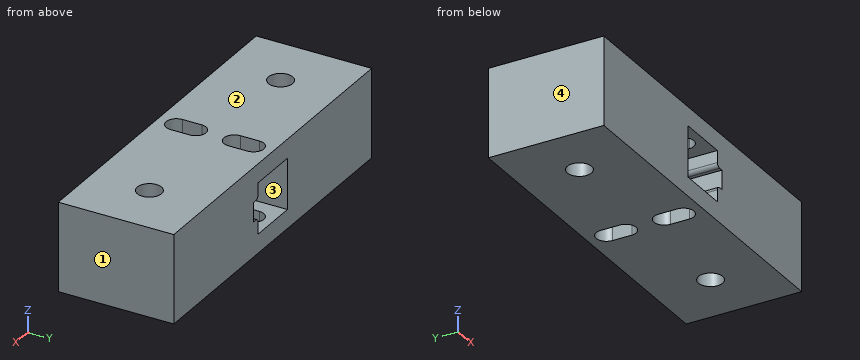
```python
from build123d import *

# Parameters (mm, degrees)
ESQUISSE1_W             = 89
ESQUISSE1_H             = 30
BOSS_EXTRU_1_DEPTH      = 23
ESQUISSE2_W             = 13.2
ESQUISSE2_H             = 13.2
ESQUISSE2_W_2           = 2
ESQUISSE2_H_2           = 5
ENL_V_MAT_EXTRU_1_DEPTH = 31
ESQUISSE3_R             = 3.15
ENL_V_MAT_EXTRU_2_DEPTH = 24
ENL_V_MAT_EXTRU_3_DEPTH = 24
CONG_1_R                = 1


with BuildPart() as part:
    # Esquisse1 → Boss.-Extru.1 (new body)
    with BuildSketch(Plane.XY):
        with Locations((40.389968792, -13.091136671)):
            Rectangle(ESQUISSE1_W, ESQUISSE1_H)
    extrude(amount=BOSS_EXTRU_1_DEPTH)

    # Esquisse2 → Enlèv. mat.-Extru.1 (cut, through all)
    with BuildSketch(Plane(origin=(0, 1.908863329, 0), x_dir=(1, 0, 0), z_dir=(0, 1, 0))):
        with Locations((40.389968792, -11.5)):
            Rectangle(ESQUISSE2_W, ESQUISSE2_H)
        with Locations((47.989968792, -11.5)):
            Rectangle(ESQUISSE2_W_2, ESQUISSE2_H_2)
    extrude(amount=-ENL_V_MAT_EXTRU_1_DEPTH, mode=Mode.SUBTRACT)

    # Esquisse3 → Enlèv. mat.-Extru.2 (cut, through all)
    with BuildSketch(Plane(origin=(0, 0, 0), x_dir=(-1, 0, 0), z_dir=(0, 0, -1))):
        with Locations((-10.889968792, -13.091136671)):
            Circle(ESQUISSE3_R)
        with Locations((-69.889968792, -13.091136671)):
            Circle(ESQUISSE3_R)
    extrude(amount=-ENL_V_MAT_EXTRU_2_DEPTH, mode=Mode.SUBTRACT)

    # Esquisse4 → Enlèv. mat.-Extru.3 (cut, through all)
    with BuildSketch(Plane(origin=(0, 0, 0), x_dir=(-1, 0, 0), z_dir=(0, 0, -1))):
        with BuildLine():
            ThreePointArc((-37.689968792, -8.091136671), (-40.389968792, -10.791136671), (-43.089968792, -8.091136671))
            Line((-43.089968792, -8.091136671), (-43.089968792, -3.091136671))
            ThreePointArc((-43.089968792, -3.091136671), (-40.389968792, -0.391136671), (-37.689968792, -3.091136671))
            Line((-37.689968792, -3.091136671), (-37.689968792, -8.091136671))
        make_face()
        with BuildLine():
            Line((-43.089968792, -23.091136671), (-43.089968792, -18.091136671))
            ThreePointArc((-43.089968792, -18.091136671), (-40.389968792, -15.391136671), (-37.689968792, -18.091136671))
            Line((-37.689968792, -18.091136671), (-37.689968792, -23.091136671))
            ThreePointArc((-37.689968792, -23.091136671), (-40.389968792, -25.791136671), (-43.089968792, -23.091136671))
        make_face()
    extrude(amount=-ENL_V_MAT_EXTRU_3_DEPTH, mode=Mode.SUBTRACT)

    # Congé1
    cong_1_edges = [part.edges().sort_by_distance(p)[0] for p in [
        (46.989968792, -13.091136671, 9),
        (46.989968792, -13.091136671, 14),
    ]]
    fillet(cong_1_edges, radius=CONG_1_R)


solid = part.part
```
Work out the finished part from the listing and answer in its coordinate system (mm). Face numbers are marked on the shaded views. Give positions to 0.01 mm unless a question says otherwise; leave off trailing zeros. Order: outer loops, then holes, each group sorted by start corner. A loop starts at its lowest first (then second) coordinate and runs counter-clockwise, first axis right, second up. Notation, with made-up numbers: (3.5, 54) - (52.5, 54) arc R8 ccw to (52.5, 62) - close; hole circle Ø8 at (25, 43.5). An arc over 180 degrees is marked (long way). One line per item, written item: value. Start each with the question number.
1. Section D-D, the plane x = 70.5 is taken. Write down the section's boundary in (y, z).
2. Section B-B, the plane x = 38.5 is taken. Write down the section's boundary in (y, z).
3. Each of these flat-tipped pins is pushed along its axis until it touches: pin 1 Ø5 at (x, y) = (10.89, -13.09) entering from +Z; pin 2 Ø10 at (x, y) = (59, -1.5) entering from -Z. Where does it stop, or does it pass through?
4. Consider line 1 (X direction, y = -12.75, z = 18.5); line 2 (X direction, y = -6, z = 2); line 3 (X direction, y = -13.25, z = 10.5). Determine where each line is inside the solid, lowest interval first.
5. Section C-C, the plane z = 10 is taken. Write down the section's boundary in (x, y).
6. Section A-A, the plane y = -20.75 is taken. Write down the section's boundary in (x, z).
7. For a pull along X with two mould halves and no side action, classify the marked faces 1, 2, 3 and 4 as released by +X, released by -X, zero draft, split by the parting line, or undercut.
Filled sheet:
1. outline: (-28.09, 0) - (-16.18, 0) - (-16.18, 23) - (-28.09, 23) - close; (-10, 0) - (1.91, 0) - (1.91, 23) - (-10, 23) - close
2. outline: (-28.09, 0) - (-25.02, 0) - (-25.02, 4.9) - (-28.09, 4.9) - close; (-28.09, 18.1) - (-25.02, 18.1) - (-25.02, 23) - (-28.09, 23) - close; (-16.16, 0) - (-10.02, 0) - (-10.02, 4.9) - (-16.16, 4.9) - close; (-16.16, 18.1) - (-10.02, 18.1) - (-10.02, 23) - (-16.16, 23) - close; (-1.16, 0) - (1.91, 0) - (1.91, 4.9) - (-1.16, 4.9) - close; (-1.16, 18.1) - (1.91, 18.1) - (1.91, 23) - (-1.16, 23) - close
3. pin 1: through
3. pin 2: z = 0
4. line 1: -4.11 to 7.76, 14.02 to 66.76, 73.02 to 84.89
4. line 2: -4.11 to 37.69, 43.09 to 84.89
4. line 3: -4.11 to 7.74, 14.04 to 33.79, 48.99 to 66.74, 73.04 to 84.89
5. outline: (-4.11, -28.09) - (33.79, -28.09) - (33.79, 1.91) - (-4.11, 1.91) - close; (48.99, -28.09) - (84.89, -28.09) - (84.89, 1.91) - (48.99, 1.91) - close; hole circle Ø6.3 at (10.89, -13.09); hole circle Ø6.3 at (69.89, -13.09)
6. outline: (-4.11, 0) - (37.69, 0) - (37.69, 4.9) - (33.79, 4.9) - (33.79, 18.1) - (37.69, 18.1) - (37.69, 23) - (-4.11, 23) - close; (43.09, 0) - (84.89, 0) - (84.89, 23) - (43.09, 23) - (43.09, 18.1) - (46.99, 18.1) - (46.99, 15) arc R1 ccw to (47.99, 14) - (48.99, 14) - (48.99, 9) - (47.99, 9) arc R1 ccw to (46.99, 8) - (46.99, 4.9) - (43.09, 4.9) - close
7. face 1: released by +X
7. face 2: zero draft
7. face 3: undercut
7. face 4: released by -X
